```python
from build123d import *

# Parameters (mm, degrees)
SKETCH_W        = 40
SKETCH_H        = 5
PAD_DEPTH       = 3
SKETCH001_R     = 2
PAD001_DEPTH    = 5
CHAMFER_SIZE    = 1
CHAMFER_FACE8_W = 40
CHAMFER_FACE8_H = 3
PAD002_DEPTH    = 2
CHAMFER001_SIZE = 2
SKETCH002_W     = 20
SKETCH002_H     = 1.5
PAD003_DEPTH    = 2


with BuildPart() as part:
    # Sketch → Pad (new body)
    with BuildSketch(Plane.XY):
        with Locations((20, 2.5)):
            Rectangle(SKETCH_W, SKETCH_H)
    extrude(amount=PAD_DEPTH)

    # Sketch001 (on Face6 of Pad) → Pad001 (join)
    with BuildSketch(Plane.XY.offset(3)):
        with Locations((5, 2.5)):
            Circle(SKETCH001_R)
        with Locations((35, 2.5)):
            Circle(SKETCH001_R)
    extrude(amount=PAD001_DEPTH)

    # Chamfer
    chamfer_edges = [part.edges().sort_by_distance(p)[0] for p in [
        (3, 2.5, 8),
        (33, 2.5, 8),
    ]]
    chamfer(chamfer_edges, length=CHAMFER_SIZE)

    # Chamfer Face8 → Pad002 (add)
    with BuildSketch(Plane(origin=(20, 5, 1.5), x_dir=(1, 0, 0), z_dir=(0, 1, 0))):
        Rectangle(CHAMFER_FACE8_W, CHAMFER_FACE8_H)
    extrude(amount=PAD002_DEPTH)

    # Chamfer001
    chamfer001_edges = [part.edges().sort_by_distance(p)[0] for p in [
        (0, 7, 1.5),
        (40, 7, 1.5),
    ]]
    chamfer(chamfer001_edges, length=CHAMFER001_SIZE)

    # Sketch002 (on Face1 of Chamfer001) → Pad003 (join)
    with BuildSketch(Plane.XY.offset(3)):
        with Locations((20, 6.25)):
            Rectangle(SKETCH002_W, SKETCH002_H)
    extrude(amount=PAD003_DEPTH)


solid = part.part
```
Geometry check sheet. Reference: the model listing, model coordinates, mm. A direction names the side the tool comes from. Give positions to 0.01 mm unless a question says otherwise; leave off trailing zeros. Order: outer loops, then holes, each group sorted by start corner. A loop starts at its lowest first (then second) coordinate and runs counter-clockwise, first axis right, second up. Notation, with made-up numbers: (17.5, -18) - (55.5, -18) arc R19 ccw to (55.5, -9) - close; hole circle Ø6 at (4.25, 64). An arc over 180 degrees is marked (long way). Write item = value, one per line. Start each with the question number.
1) Access from +Z, -Z, +X, -X, +Y, -Y to the whole of each face (thin tool, end or side, straight path). Record for faces 4 (the flat face through (20, 5.5, 4)), 5 (the cylindrical face through (3.002, 2.588, 4.972)), 6 (the flat face through (39, 6, 2)).
2) Scan lines: L1, parallel to Z at x = 18, y = 3.25; L2, parallel to Z at x = 26, y = 6; L3, parallel to X at y = 4.25, z = 4.75. Record each from-to range of solid material in increasing order.
3) Section check C-C (z = 6). Enter the section's corners in (x, y), then the cut area to 3 significant figures.
4) Section check A-A (x = 35). Enter the section's corners in (y, z), then the cut area to 3 significant figures.
5) Draft check along X on faces 1 (the flat face through (10, 6, 4)), 2 (the flat face through (30, 6, 4)), 3 (the cylindrical face through (36.847, 1.734, 4.972)). Enter one of: released by +X, released by -X, zero draft, split by the parting line, or undercut.
6) Gauge pin test, flat ends, axial feed: pin 1 Ø2 at (x, y) = (13, 2.5) entering from -Z; pin 2 Ø0.8 at (x, y) = (15, 6.5) entering from +Z; pin 3 Ø1.2 at (y, z) = (6.5, 4) entering from -X; pin 4 Ø0.6 at (x, z) = (25, 4.5) entering from -Y. Record the tip position at first contact, or that the pin passes through.
7) Section check B-B (y = 2.5). Enter the section's corners in (x, z), then the cut area to 3 significant figures.
8) Section check D-D (x = 16). Enter the section's corners in (y, z).
Geometry check:
q1.face_4 = +Z, +X, -X, -Y
q1.face_5 = +Z
q1.face_6 = +Z, -Z, +X, +Y
q2.L1 = 0 to 3
q2.L2 = 0 to 5
q2.L3 = 4.03 to 5.97, 34.03 to 35.97
q3.outline = circle Ø4 at (5, 2.5); circle Ø4 at (35, 2.5)
q3.area = 25.1 mm2
q4.outline = (0, 0) - (7, 0) - (7, 3) - (4.5, 3) - (4.5, 7) - (3.5, 8) - (1.5, 8) - (0.5, 7) - (0.5, 3) - (0, 3) - close
q4.area = 40.0 mm2
q5.face_1 = released by -X
q5.face_2 = released by +X
q5.face_3 = undercut
q6.pin_1 = 0
q6.pin_2 = 5
q6.pin_3 = 10
q6.pin_4 = 5.5
q7.outline = (0, 0) - (40, 0) - (40, 3) - (37, 3) - (37, 7) - (36, 8) - (34, 8) - (33, 7) - (33, 3) - (7, 3) - (7, 7) - (6, 8) - (4, 8) - (3, 7) - (3, 3) - (0, 3) - close
q7.area = 158 mm2
q8.outline = (0, 0) - (7, 0) - (7, 5) - (5.5, 5) - (5.5, 3) - (0, 3) - close
